Read the model definition and answer for the solid it produces. Units are mm, in the model's axes. Face numbers are marked on the shaded views. Round coordinates to 2 decimals unless told otherwise and drop trailing zeros. Write each loop counter-clockwise with the first axis right and the second up, starting at its lowest first coordinate (ties: lowest second). Pieces come first, ordered by that corner, then holes.
from build123d import *

# Parameters (mm, degrees)
SKETCH1_W           = 110
SKETCH1_H           = 110
BOSS_EXTRUDE1_DEPTH = 4
SKETCH2_W           = 80
SKETCH2_H           = 80
SKETCH2_W_2         = 60
SKETCH2_H_2         = 60
BOSS_EXTRUDE2_DEPTH = 9.525
SKETCH3_R           = 24.000000006
CUT_EXTRUDE1_DEPTH  = 20


with BuildPart() as part:
    # Sketch1 → Boss-Extrude1 (new body)
    with BuildSketch(Plane(origin=(0, 0, 0), x_dir=(1, 0, 0), z_dir=(0, 1, 0))):
        Rectangle(SKETCH1_W, SKETCH1_H)
    extrude(amount=-BOSS_EXTRUDE1_DEPTH)

    # Sketch2 → Boss-Extrude2 (add)
    with BuildSketch(Plane(origin=(0, 0, 0), x_dir=(1, 0, 0), z_dir=(0, 1, 0))):
        Rectangle(SKETCH2_W, SKETCH2_H)
        Rectangle(SKETCH2_W_2, SKETCH2_H_2, mode=Mode.SUBTRACT)
    extrude(amount=BOSS_EXTRUDE2_DEPTH)

    # Sketch3 → Cut-Extrude1 (cut)
    with BuildSketch(Plane(origin=(0, 0, 0), x_dir=(1, 0, 0), z_dir=(0, 1, 0))):
        with Locations(Location((0, 0, 0), (0, 0, 270))):
            Circle(SKETCH3_R)
    extrude(amount=-CUT_EXTRUDE1_DEPTH, mode=Mode.SUBTRACT)


solid = part.part
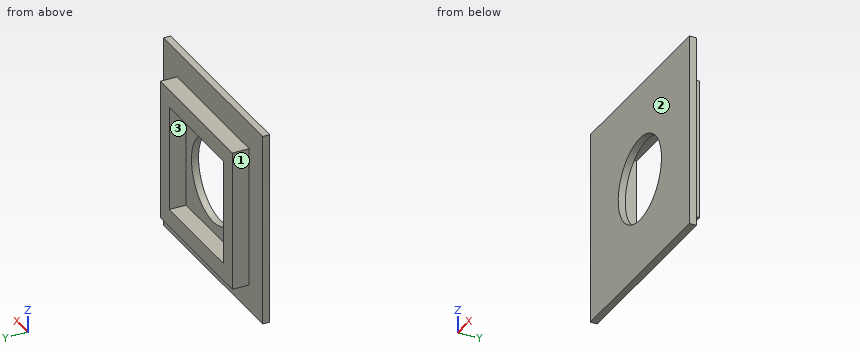
Q1. Section D-D (x = -28) is taken. Determine the outline of the cut face in (y, z) (3 decimals).
Verdict:
outline: (-4, -55) - (0, -55) - (0, -40) - (9.525, -40) - (9.525, -30) - (0, -30) - (0, 30) - (9.525, 30) - (9.525, 40) - (0, 40) - (0, 55) - (-4, 55) - close
Q2. Determine the mould class of the marked faces 1, 2 and 3 for opening direction X: pulls with the +X half, pulls with the -X half, needs draft (parallel to the pull), parting line crosses it, or undercut.
Verdict:
face 1: pulls with the -X half
face 2: needs draft
face 3: undercut
Q3. Flat-ended cylindrical pins translate along their axes: pin 1 Ø5 at (y, z) = (5, -5) entering from -X; pin 2 Ø5 at (x, y) = (15, 5) entering from +Z; pin 3 Ø7.5 at (x, y) = (0, 4) entering from -Z; pin 4 Ø1 at (x, z) = (-13.5, 18) entering from +Y. Find the tip coordinate at first contact, or state that the pin passes through.
Verdict:
pin 1: stops at x = -40
pin 2: stops at z = 40
pin 3: stops at z = -40
pin 4: passes through
Q4. Section A-A (x = 0) is taken. Determine the outline of the cut face in (y, z) (3 decimals), then the cut area to 4 significant figures.
Verdict:
outline: (-4, -55) - (0, -55) - (0, -40) - (9.525, -40) - (9.525, -30) - (0, -30) - (0, -24) - (-4, -24) - close; (-4, 24) - (0, 24) - (0, 30) - (9.525, 30) - (9.525, 40) - (0, 40) - (0, 55) - (-4, 55) - close
area: 438.5 mm2
Q5. Section C-C (y = 4.75) is taken. Determine the outline of the cut face in (x, z).
Verdict:
outline: (-40, -40) - (40, -40) - (40, 40) - (-40, 40) - close; hole (-30, -30) - (30, -30) - (30, 30) - (-30, 30) - close
Q6. Section B-B (z = 0) is taken. Determine the outline of the cut face in (x, y) (3 decimals), then the cut area to 4 significant figures.
Verdict:
outline: (-55, -4) - (-24, -4) - (-24, 0) - (-30, 0) - (-30, 9.525) - (-40, 9.525) - (-40, 0) - (-55, 0) - close; (24, -4) - (55, -4) - (55, 0) - (40, 0) - (40, 9.525) - (30, 9.525) - (30, 0) - (24, 0) - close
area: 438.5 mm2
Q7. Straight lines are drawn through the part: probe 1 along Z at (x, y) = (16, 4.5); probe 2 along X at (y, z) = (-2.75, 0); probe 3 along Y at (x, z) = (-5, 43). For each, find the intervals that lie inside material, in ascending order.
Verdict:
probe 1: z = -40 to -30, 30 to 40
probe 2: x = -55 to -24, 24 to 55
probe 3: y = -4 to 0
